```python
from build123d import *

# Parameters (mm, degrees)
SKETCH1_W           = 38.1
SKETCH1_H           = 76.2
BOSS_EXTRUDE1_DEPTH = 2.54
SKETCH1_3_R         = 9.549995
SKETCH1_3_R_2       = 7.05
BOSS_EXTRUDE2_DEPTH = 7.62
FILLET1_R           = 1.27


with BuildPart() as part:
    # Sketch1 → Boss-Extrude1 (new body)
    with BuildSketch(Plane(origin=(0, 0, 0), x_dir=(1, 0, 0), z_dir=(0, 1, 0))):
        with Locations((19.05, 38.1)):
            Rectangle(SKETCH1_W, SKETCH1_H)
    extrude(amount=BOSS_EXTRUDE1_DEPTH)

    # Sketch1_3 → Boss-Extrude2 (add)
    with BuildSketch(Plane(origin=(0, 0, 0), x_dir=(1, 0, 0), z_dir=(0, 1, 0))):
        with Locations(Location((19.05, 12.7, 0), (0, 0, 270))):
            Circle(SKETCH1_3_R)
        with Locations(Location((19.05, 12.7, 0), (0, 0, 270))):
            Circle(SKETCH1_3_R_2, mode=Mode.SUBTRACT)
    extrude(amount=-BOSS_EXTRUDE2_DEPTH)

    # Fillet1
    fillet1_edges = [part.edges().sort_by_distance(p)[0] for p in [
        (19.05, 0, -22.249995),
        (0, 1.27, 0),
        (38.1, 1.27, 0),
    ]]
    fillet(fillet1_edges, radius=FILLET1_R)


solid = part.part
```
Check sheet for the modelled part. Datum: model origin and axes. Units: mm. A direction names the side the tool comes from. Coordinates: 2 decimals unless noted, no trailing zeros. Write each loop counter-clockwise with the first axis right and the second up, starting at its lowest first coordinate (ties: lowest second). Pieces come first, ordered by that corner, then holes. Notation, with made-up numbers: (81.5, 76.25) -> (139.5, 76.25) arc R21 ccw to (139.5, 105.25) -> close; hole circle Ø10 at (70.25, -23.5). An arc over 180 degrees is marked (long way). Use a Markdown table: item, result.
1. Sectioned sample at C-C (x = 19.05). Enter the section's corners in (y, z).
Reported:
| item | result |
|---|---|
| outline | (-7.62, -22.25) -> (-1.27, -22.25) arc R1.27 cw to (0, -23.52) -> (0, -76.2) -> (2.54, -76.2) -> (2.54, 0) -> (0, 0) -> (0, -1.88) arc R1.27 cw to (-1.27, -3.15) -> (-7.62, -3.15) -> (-7.62, -5.65) -> (0, -5.65) -> (0, -19.75) -> (-7.62, -19.75) -> close |
2. Release check for a two-part mould opening along X. For faces 3 (the flat face through (19, 1, 0)), 4 (the flat face through (0, 1, -38)), 5 (the cylindrical face through (12.795, -3.757, -9.447)) record: pulls with the +X half, pulls with the -X half, needs draft (parallel to the pull), parting line crosses it, or undercut.
Reported:
| item | result |
|---|---|
| face 3 | needs draft |
| face 4 | pulls with the -X half |
| face 5 | undercut |
3. Tool access check on faces 1 (the flat face through (19, 0, -13)), 2 (the flat face through (19, 1, -76.2)). Record the directions out of +Z, -Z, +X, -X, +Y, -Y that give a thin tool (end or side, any length) a straight path to the whole face; none if there is none.
Reported:
| item | result |
|---|---|
| face 1 | -Y |
| face 2 | -Z, +X, -X, +Y, -Y |
4. Sectioned sample at B-B (y = -4.5). Enter the section's corners in (x, z), plus the area to 3 significant figures.
Reported:
| item | result |
|---|---|
| outline | circle Ø19.1 at (19.05, -12.7); hole circle Ø14.1 at (19.05, -12.7) |
| area | 130 mm2 |
5. Scan lines: line 1 along X through (y, z) = (-3.75, -12.7); line 2 along Y through (x, z) = (26, -64); line 3 along X through (y, z) = (-4.75, -7). Record each from-to range of solid material in increasing order.
Reported:
| item | result |
|---|---|
| line 1 | x = 9.5 to 12, 26.1 to 28.6 |
| line 2 | y = 0 to 2.54 |
| line 3 | x = 11.39 to 14.9, 23.2 to 26.71 |
6. Go/stop test with flat-tipped pins: pin 1 Ø3 at (x, z) = (25, -31) entering from -Y; pin 2 Ø1 at (x, y) = (14.5, -4) entering from +Z; pin 3 Ø5 at (y, z) = (-4.5, -43.5) entering from -X; pin 4 Ø11.5 at (x, z) = (21, -10) entering from -Y. Record where each tip stops, or that it passes through.
Reported:
| item | result |
|---|---|
| pin 1 | stops at y = 0 |
| pin 2 | stops at z = -4.05 |
| pin 3 | passes through |
| pin 4 | stops at y = -7.62 |
7. Sectioned sample at D-D (x = 3). Enter the section's corners in (y, z).
Reported:
| item | result |
|---|---|
| outline | (0, -76.2) -> (2.54, -76.2) -> (2.54, 0) -> (0, 0) -> close |
8. Sectioned sample at A-A (z = -12.7). Enter the section's corners in (x, y).
Reported:
| item | result |
|---|---|
| outline | (0, 0) -> (8.23, 0) arc R1.27 cw to (9.5, -1.27) -> (9.5, -7.62) -> (12, -7.62) -> (12, 0) -> (26.1, 0) -> (26.1, -7.62) -> (28.6, -7.62) -> (28.6, -1.27) arc R1.27 cw to (29.87, 0) -> (38.1, 0) -> (38.1, 2.54) -> (0, 2.54) -> close |
